Geometry: final body of the model. Coordinates: model frame, mm. A direction names the side the tool comes from. Give positions to 0.01 mm unless a question says otherwise; leave off trailing zeros.
```python
from build123d import *

# Parameters (mm, degrees)
F1_DEPTH = 6.35


with BuildPart() as f1:
    # F0 (on Top) → F1 (new body)
    with BuildSketch(Plane.XY):
        with BuildLine():
            add(Edge.make_bspline(
                [(-4.167193, 43.824071), (-7.616309, 43.824071), (-10.412782, 41.148246), (-10.412782, 37.848004)],
                knots=[0, 0, 0, 0, 1, 1, 1, 1], degree=3))
            Line((-10.412782, 37.848004), (-10.412782, 36.849643))
            Line((-10.412782, 36.849643), (-14.572746, 36.849643))
            add(Edge.make_bspline(
                [(-14.572746, 36.849643), (-18.021507, 36.849643), (-20.817982, 34.174171), (-20.817982, 30.873929)],
                knots=[0, 0, 0, 0, 1, 1, 1, 1], degree=3))
            Line((-20.817982, 30.873929), (-20.817982, -30.878161))
            add(Edge.make_bspline(
                [(-20.817982, -30.878161), (-20.817982, -34.178759), (-18.021507, -36.854228), (-14.572746, -36.854228)],
                knots=[0, 0, 0, 0, 1, 1, 1, 1], degree=3))
            Line((-14.572746, -36.854228), (-10.412782, -36.854228))
            Line((-10.412782, -36.854228), (-10.412782, -37.848356))
            add(Edge.make_bspline(
                [(-10.412782, -37.848356), (-10.412782, -41.148598), (-7.616309, -43.82407), (-4.167193, -43.82407)],
                knots=[0, 0, 0, 0, 1, 1, 1, 1], degree=3))
            Line((-4.167193, -43.82407), (4.160141, -43.82407))
            add(Edge.make_bspline(
                [(4.160141, -43.82407), (7.609255, -43.82407), (10.405374, -41.148598), (10.405374, -37.848356)],
                knots=[0, 0, 0, 0, 1, 1, 1, 1], degree=3))
            Line((10.405374, -37.848356), (10.405374, -36.854228))
            Line((10.405374, -36.854228), (14.572747, -36.854228))
            add(Edge.make_bspline(
                [(14.572747, -36.854228), (18.021861, -36.854228), (20.817983, -34.178759), (20.817983, -30.878161)],
                knots=[0, 0, 0, 0, 1, 1, 1, 1], degree=3))
            Line((20.817983, -30.878161), (20.817983, 30.873929))
            add(Edge.make_bspline(
                [(20.817983, 30.873929), (20.817983, 34.174171), (18.021861, 36.849643), (14.572747, 36.849643)],
                knots=[0, 0, 0, 0, 1, 1, 1, 1], degree=3))
            Line((14.572747, 36.849643), (10.405374, 36.849643))
            Line((10.405374, 36.849643), (10.405374, 37.848004))
            add(Edge.make_bspline(
                [(10.405374, 37.848004), (10.405374, 41.148246), (7.609255, 43.824071), (4.160141, 43.824071)],
                knots=[0, 0, 0, 0, 1, 1, 1, 1], degree=3))
            Line((4.160141, 43.824071), (-4.167193, 43.824071))
        make_face()
    extrude(amount=F1_DEPTH)


solid = f1.part
```
Q1. Pin query (flat end, axial travel): pin 1 Ø1.5 at (x, z) = (-8.5, 2) entering from -Y; pin 2 Ø2 at (x, z) = (-13.5, 3) entering from -Y; pin 3 Ø1.1 at (y, z) = (37.5, 2.5) entering from +X; pin 4 Ø10 at (x, y) = (-1, 33) entering from -Z. Return the tip coordinate at first contact, or that it passes through.
Q2. Material intervals for probe 1 along Y at (x, z) = (11.5, 1); probe 2 along X at (y, z) = (-37, 5.75); probe 3 along Y at (x, z) = (9.5, 5), sorted ascending.
Q3. Reachability of faces 1 (the face through (-12, 36.85, 3)), 2 (the face through (13, 36.85, 3)), 3 (the face through (12, -36.854, 3)), 4 (the face through (0, 1, 0)), 5 (the face through (-13, -36.854, 3)) from +Z, -Z, +X, -X, +Y, -Y: full face, straight path, thin tool, end or side. Return the list, or none.
Resolved:
1. pin 1: stops at y = -42.74
1. pin 2: stops at y = -36.85
1. pin 3: stops at x = 10.41
1. pin 4: stops at z = 0
2. probe 1: y = -36.85 to 36.85
2. probe 2: x = -10.41 to 10.41
2. probe 3: y = -40.95 to 40.95
3. face 1: +Z, -Z, -X, +Y
3. face 2: +Z, -Z, +X, +Y
3. face 3: +Z, -Z, +X, -Y
3. face 4: -Z, +X, -X, +Y, -Y
3. face 5: +Z, -Z, -X, -Y
